from build123d import *

# Parameters (mm, degrees)
EXTRUDE_1_DEPTH     = 30
CUT_EXTRUDE_1_REACH = 59.879
SKETCH_2_R          = 1.5
SKETCH_2_W          = 30
SKETCH_2_H          = 10
SKETCH_3_R          = 2.1
CUT_EXTRUDE_2_DEPTH = 53.440442409
SKETCH_4_W          = 30
SKETCH_4_H          = 3
CUT_EXTRUDE_3_DEPTH = 13


with BuildPart() as part:
    # 草图1 → 凸台-拉伸1 (new body)
    with BuildSketch(Plane(origin=(0, 0, 0), x_dir=(0, 0, -1), z_dir=(1, 0, 0))):
        Polygon((0, 0), (0, 35), (3, 35), (3, -3), (-35, -3), (-35, 0), align=None)
    extrude(amount=EXTRUDE_1_DEPTH)

    # 草图2 → 切除-拉伸1 (cut, up to next)
    with BuildSketch(Plane(origin=(0, 0, 0), x_dir=(1, 0, 0), z_dir=(0, 1, 0)), mode=Mode.PRIVATE) as cut_extrude_1_sk1:
        with Locations(Location((9, -7, 0), (0, 0, 270))):
            Circle(SKETCH_2_R)
    cut_extrude_1_tool1 = extrude(cut_extrude_1_sk1.sketch, amount=-CUT_EXTRUDE_1_REACH, mode=Mode.PRIVATE) & part.part
    # 草图2 → 切除-拉伸1 (cut, up to next)
    with BuildSketch(Plane(origin=(0, 0, 0), x_dir=(1, 0, 0), z_dir=(0, 1, 0)), mode=Mode.PRIVATE) as cut_extrude_1_sk2:
        with Locations(Location((9, -19, 0), (0, 0, 270))):
            Circle(SKETCH_2_R)
    cut_extrude_1_tool2 = extrude(cut_extrude_1_sk2.sketch, amount=-CUT_EXTRUDE_1_REACH, mode=Mode.PRIVATE) & part.part
    # 草图2 → 切除-拉伸1 (cut, up to next)
    with BuildSketch(Plane(origin=(0, 0, 0), x_dir=(1, 0, 0), z_dir=(0, 1, 0)), mode=Mode.PRIVATE) as cut_extrude_1_sk3:
        with Locations(Location((21, -19, 0), (0, 0, 270))):
            Circle(SKETCH_2_R)
    cut_extrude_1_tool3 = extrude(cut_extrude_1_sk3.sketch, amount=-CUT_EXTRUDE_1_REACH, mode=Mode.PRIVATE) & part.part
    # 草图2 → 切除-拉伸1 (cut, up to next)
    with BuildSketch(Plane(origin=(0, 0, 0), x_dir=(1, 0, 0), z_dir=(0, 1, 0)), mode=Mode.PRIVATE) as cut_extrude_1_sk4:
        with Locations(Location((21, -7, 0), (0, 0, 270))):
            Circle(SKETCH_2_R)
    cut_extrude_1_tool4 = extrude(cut_extrude_1_sk4.sketch, amount=-CUT_EXTRUDE_1_REACH, mode=Mode.PRIVATE) & part.part
    # 草图2 → 切除-拉伸1 (cut, up to next)
    with BuildSketch(Plane(origin=(0, 0, 0), x_dir=(1, 0, 0), z_dir=(0, 1, 0)), mode=Mode.PRIVATE) as cut_extrude_1_sk5:
        with Locations((15, -30)):
            Rectangle(SKETCH_2_W, SKETCH_2_H)
    cut_extrude_1_tool5 = extrude(cut_extrude_1_sk5.sketch, amount=-CUT_EXTRUDE_1_REACH, mode=Mode.PRIVATE) & part.part
    add(cut_extrude_1_tool1.solids().sort_by_distance((9, 0, 7))[0], mode=Mode.SUBTRACT)
    add(cut_extrude_1_tool2.solids().sort_by_distance((9, 0, 19))[0], mode=Mode.SUBTRACT)
    add(cut_extrude_1_tool3.solids().sort_by_distance((21, 0, 19))[0], mode=Mode.SUBTRACT)
    add(cut_extrude_1_tool4.solids().sort_by_distance((21, 0, 7))[0], mode=Mode.SUBTRACT)
    add(cut_extrude_1_tool5.solids().sort_by_distance((15, 0, 30))[0], mode=Mode.SUBTRACT)

    # 草图3 → 切除-拉伸2 (cut, through all)
    with BuildSketch(Plane.XY):
        with Locations((15, 23.25)):
            Circle(SKETCH_3_R)
    extrude(amount=-CUT_EXTRUDE_2_DEPTH, mode=Mode.SUBTRACT)

    # 草图4 → 切除-拉伸3 (cut)
    with BuildSketch(Plane.XY.offset(25)):
        with Locations((15, -1.5)):
            Rectangle(SKETCH_4_W, SKETCH_4_H)
    extrude(amount=-CUT_EXTRUDE_3_DEPTH, mode=Mode.SUBTRACT)


solid = part.part
Work out the finished part from the listing and answer in its coordinate system (mm). A direction names the side the tool comes from. Round coordinates to 2 decimals unless told otherwise and drop trailing zeros. Order: outer loops, then holes, each group sorted by start corner. A loop starts at its lowest first (then second) coordinate and runs counter-clockwise, first axis right, second up. Notation, with made-up numbers: M 35.5,-0.5 L 92.5,-0.5 A28 ccw 92.5,32.5 Z; hole C -11,-15.5 d10. An arc over 180 degrees is marked long. One line per item, written item: value.
Q1. Find section B-B on y = 23.25. Write down the section's boundary in (x, z), then the cut area to 3 significant figures.
Derived:
outline: M 0,-3 L 12.9,-3 L 12.9,0 L 0,0 Z; M 17.1,-3 L 30,-3 L 30,0 L 17.1,0 Z
area: 77.4 mm²
Q2. Straight lines are drawn through the part: line 1 (X direction, y = -2.3, z = 7); line 2 (Y direction, x = 15, z = -0.8); line 3 (Z direction, x = 11.25, y = 24). For each, find the intervals that lie inside material, in ascending order.
Derived:
line 1: 0 to 7.5, 10.5 to 19.5, 22.5 to 30
line 2: -3 to 21.15, 25.35 to 35
line 3: -3 to 0
Q3. Find section C-C on x = 9. Write down the section's boundary in (y, z).
Derived:
outline: M -3,-3 L 35,-3 L 35,0 L 0,0 L 0,5.5 L -3,5.5 Z; M -3,8.5 L 0,8.5 L 0,12 L -3,12 Z
Q4. For faces 1 (the face through (30, 12, -1)), 2 (the face through (15, 17, 0)), determine the directions among +Z, -Z, +X, -X, +Y, -Y from which every point of the face is accessible in a straight line to the end or side of a thin tool.
Derived:
face 1: +Z, -Z, +X, +Y, -Y
face 2: +Z, +X, -X, +Y
Q5. Flat-ended cylindrical pins translate along their axes: pin 1 (6 mm diameter, centred on x = 12, y = 14.5, fed in from +Z); pin 2 (2.5 mm diameter, centred on x = 21, z = 7, fed in from +Y); pin 3 (6 mm diameter, centred on x = 23.5, z = 6.5, fed in from +Y). Find the tip coordinate at first contact, or state that the pin passes through.
Derived:
pin 1: z = 0
pin 2: through
pin 3: y = 0
Q6. Determine the mould class of faces 3 (the face through (15, 35, -1)), 4 (the face through (8.1, -1.5, 5.8)), 5 (the face through (0, 12, -1)), 6 (the face through (22.01, -1.48, 5.89)) for opening direction X: released by +X, released by -X, zero draft, split by the parting line, or undercut.
Derived:
face 3: zero draft
face 4: undercut
face 5: released by -X
face 6: undercut
Q7. Find section A-A on z = 7. Write down the section's boundary in (x, y).
Derived:
outline: M 0,-3 L 7.5,-3 L 7.5,0 L 0,0 Z; M 10.5,-3 L 19.5,-3 L 19.5,0 L 10.5,0 Z; M 22.5,-3 L 30,-3 L 30,0 L 22.5,0 Z
Q8. Find section D-D on x = 24.25. Write down the section's boundary in (y, z), then the cut area to 3 significant figures.
Derived:
outline: M -3,-3 L 35,-3 L 35,0 L 0,0 L 0,12 L -3,12 Z
area: 150 mm²
